Read the model definition and answer for the solid it produces. Units are mm, in the model's axes. A direction names the side the tool comes from. Round coordinates to 2 decimals unless told otherwise and drop trailing zeros. Loops run counter-clockwise (first coordinate to the right, second up) from the corner with the lowest first, then second, coordinate; pieces in that order, holes last. Notation, with made-up numbers: M -28,-25.75 L -10,-25.75 A17 cw -10,-11.75 Z; hole C 44,40 d7. An arc over 180 degrees is marked long. Write each question's results on one line, items separated by ' | '.
```python
from build123d import *

# Parameters (mm, degrees)
EXTRUDE1_DEPTH             = 130
FILLET1_R                  = 25
EXTRUDE2_DEPTH             = 130
SKETCH3_W                  = 45
SKETCH3_H                  = 25
EXTRUDE3_DEPTH             = 5
SKETCH4_W                  = 80
SKETCH4_H                  = 30
EXTRUDE4_DEPTH             = 40
SKETCH5_R                  = 22
EXTRUDE5_DEPTH             = 40
EXTRUDE5_DIRECTION_2_REACH = 77


with BuildPart() as part:
    # Sketch1 → Extrude1 (new body)
    with BuildSketch(Plane(origin=(0, 0, 0), x_dir=(0, 0, -1), z_dir=(1, 0, 0))):
        Polygon((0, 0), (0, 110), (-25, 110), (-61, 62), (-75, 62), (-105, 22), (-140, 22), (-140, 17), (-105, 0), align=None)
    extrude(amount=EXTRUDE1_DEPTH)

    # Fillet1
    fillet1_edges = [part.edges().sort_by_distance(p)[0] for p in [
        (0, 55, 0),
        (130, 55, 0),
    ]]
    fillet(fillet1_edges, radius=FILLET1_R)

    # Sketch2 → Extrude2 (cut)
    with BuildSketch(Plane(origin=(0, 22, 0), x_dir=(1, 0, 0), z_dir=(0, 1, 0))):
        Polygon((99.792740578, -140), (130, -140), (130, -105), (120, -105), align=None)
        Polygon((10, -105), (30.207259422, -140), (0, -140), (0, -105), align=None)
    extrude(amount=-EXTRUDE2_DEPTH, mode=Mode.SUBTRACT)

    # Sketch3 → Extrude3 (cut)
    with BuildSketch(Plane(origin=(130, 0, 0), x_dir=(0, 0, -1), z_dir=(1, 0, 0))):
        with Locations((-47.5, 34.5)):
            Rectangle(SKETCH3_W, SKETCH3_H)
    extrude(amount=-EXTRUDE3_DEPTH, mode=Mode.SUBTRACT)

    # Sketch4 → Extrude4 (cut)
    with BuildSketch(Plane(origin=(0, 62, 0), x_dir=(1, 0, 0), z_dir=(0, 1, 0))):
        with Locations((65, -90)):
            Rectangle(SKETCH4_W, SKETCH4_H)
    extrude(amount=-EXTRUDE4_DEPTH, mode=Mode.SUBTRACT)

    # Sketch5 → Extrude5 (add)
    with BuildSketch(Plane.XY.offset(75)):
        with Locations((65, 62)):
            Circle(SKETCH5_R)
    extrude(amount=EXTRUDE5_DEPTH)

    # Extrude5 direction 2: up to this face of the body (flat: up to its plane)
    extrude5_direction_2_end = Plane(part.part.faces().sort_by_distance((65, 86, 43))[0])
    # Sketch5 → Extrude5 direction 2 (add, up to the picked face)
    with BuildSketch(Plane.XY.offset(75), mode=Mode.PRIVATE) as extrude5_direction_2_sk1:
        with Locations((65, 62)):
            Circle(SKETCH5_R)
    extrude5_direction_2_tool1 = split(extrude(extrude5_direction_2_sk1.sketch, amount=-EXTRUDE5_DIRECTION_2_REACH, mode=Mode.PRIVATE), bisect_by=extrude5_direction_2_end, keep=Keep.BOTH, mode=Mode.PRIVATE)
    add(extrude5_direction_2_tool1.solids().sort_by(Axis((65, 62, 75), (0, 0, -1)))[0])


solid = part.part
```
1. Find the intervals of material crossed by L1, parallel to X at y = 29.5, z = 93; L2, parallel to Z at x = 90, y = 33.5; L3, parallel to Z at x = 52, y = 54.5, in increasing order.
Completed:
L1: x = 0 to 25, 105 to 130 | L2: z = 0 to 75 | L3: z = 0 to 115
2. Find section C-C, the plane y = 34. Give the vertices of the cut face in (x, z), then the cut area to 3 significant figures.
Completed:
outline: M 0,25 A25 ccw 25,0 L 105,0 A25 ccw 130,25 L 125,25 L 125,70 L 130,70 L 130,96 L 105,96 L 105,75 L 25,75 L 25,96 L 0,96 Z | area: 10,300 mm2
3. Find section D-D, the plane z = 55. Give the vertices of the cut face in (x, y).
Completed:
outline: M 0,0 L 130,0 L 130,22 L 125,22 L 125,47 L 130,47 L 130,70 L 85.49,70 A22 ccw 44.51,70 L 0,70 Z
4. Which of the six approach directions +Z, -Z, +X, -X, +Y, -Y give full straight-line access (tool end or side, diameter ignored) to faces 5 (the face through (12, 42, 90)), 6 (the face through (105, 33, 84)), 7 (the face through (128, 22, 48))?
Completed:
face 5: +Z, -X, +Y | face 6: +Z, +Y | face 7: +X
5. Given P1, Ø2, axis at y = 53, z = 85, coming from the +X side; P2, Ø20, axis at y = 39.5, z = 38, coming from the +X side; P3, Ø4, axis at x = 116.5, z = 67.5, coming from the +Y side; P4, Ø6, axis at x = 18, y = 64.5, coming from the +Z side (3 decimals), each flat-ended and moving along its own axis, determine where each tip first touches the part or whether it passes through.
Completed:
P1: stops at x = 85.49 | P2: stops at x = 130 | P3: stops at y = 62 | P4: stops at z = 75.375
6. Determine the mould class of faces 1 (the face through (64, 22, 107)), 2 (the face through (128, 34, 25)), 3 (the face through (117, 42, 90)), 4 (the face through (65, 20, 140)) for opening direction Y: released by +Y, released by -Y, zero draft, split by the parting line, or undercut.
Completed:
face 1: undercut | face 2: undercut | face 3: released by +Y | face 4: zero draft
7. Find section A-A, the plane x = 65. Give the vertices of the cut face in (y, z), then the cut area to 3 significant figures.
Completed:
outline: M 0,0 L 110,0 L 110,25 L 84,44.5 L 84,115 L 40,115 L 40,75 L 22,75 L 22,140 L 17,140 L 0,105 Z | area: 10,100 mm2
8. Find section B-B, the plane z = 98. Give the vertices of the cut face in (x, y), then the cut area to 3 significant figures.
Completed:
outline: M 0,0 L 130,0 L 130,31.33 L 105,31.33 L 105,22 L 25,22 L 25,31.33 L 0,31.33 Z; C 65,62 d44 | area: 4,850 mm2
